Source: CAD feature listing. Evaluate the final solid. Frame: model axes, mm. Coordinates: 2 decimals unless noted, no trailing zeros. Write each loop counter-clockwise with the first axis right and the second up, starting at its lowest first coordinate (ties: lowest second). Pieces come first, ordered by that corner, then holes. Notation, with made-up numbers: (-21, 41.5) -> (36, 41.5) arc R12 cw to (36, 51.5) -> close; hole circle Ø3 at (49.5, 80.5). An arc over 180 degrees is marked (long way). One line per item, written item: value. Start each with the question number.
1. Line query: line 1 (X direction, y = 1014, z = 7.25); line 2 (Y direction, x = -143.5, z = 4.75); line 3 (Y direction, x = -800, z = 6). Output: solid intervals per line, ascending.
2. Section query C-C, the plane x = -800. Output: boundary loops of the cut face in (y, z).
3. Section query D-D, the plane x = -462. Output: boundary loops of the cut face in (y, z), and give its area (3 significant figures).
4. Section query A-A, the plane y = 80. Output: boundary loops of the cut face in (x, z).
5. Section query B-B, the plane z = 1.5. State how many separate pieces and enclosed holes the cut face has, and give its area (3 significant figures).
Autodesk Inventor part; units mm, degrees
ref_plane "YZ Plane" through (0, 0, 0) normal (1, 0, 0) x (0, 1, 0)
ref_plane "XZ Plane" through (0, 0, 0) normal (0, 1, 0) x (-1, 0, 0)
ref_plane "XY Plane" through (0, 0, 0) normal (0, 0, 1) x (1, 0, 0)
sketch "Sketch1" plane through (0, 0, 0) normal (0, 0, 1) x (1, 0, 0)
  line L0 (0, 0) -> (0, 1910) construction
  line L1 (424.5155, 1910) -> (-415.4845, 1910)
  line L2 (-415.4845, 1910) -> (-1180, 1150)
  line L3 (-1180, 0) -> (-1180, 1150)
  line L4 (960, 0) -> (960, 1342.8524)
  line L5 (424.5155, 1910) -> (960, 1342.8524)
  circle A0 centre (0, 950) radius 265 construction
  line L6 (960, 0) -> (-1180, 0)
  circle A1 centre (-1701.6377, -269.2167) radius 188.5 construction
  circle A2 centre (-800, 80) radius 55.5
  circle A3 centre (0, 950) radius 170
  line L7 (0, 1215) -> (0, 1120) construction
  line L8 (-721.2646, 955) -> (721.2646, 955) construction
  line L9 (-169.9265, 955) -> (-174.9265, 955) construction
  line L10 (-174.9265, 960) -> (-174.9265, 950)
  line L11 (-174.9265, 960) -> (-169.7056, 960)
  line L12 (-174.9265, 950) -> (-170, 950)
  line L13 (169.9265, 955) -> (174.9265, 955) construction
  line L14 (174.9265, 960) -> (174.9265, 950)
  line L15 (169.7056, 960) -> (174.9265, 960)
  line L16 (174.9265, 950) -> (170, 950)
  line L17 (-174.9265, 970) -> (174.9265, 970)
  line L18 (174.9265, 970) -> (174.9265, 940)
  line L19 (174.9265, 940) -> (-174.9265, 940)
  line L20 (-174.9265, 940) -> (-174.9265, 970)
  arc A4 (-2.4999, 780.0184) -> (2.4999, 780.0184) centre (0, 780) ccw
  arc A5 (2.4999, 1119.9816) -> (-2.4999, 1119.9816) centre (0, 1120) ccw
  point P0 (0, 955)
  point P1 (-169.7056, 940)
  point P2 (169.7056, 940)
  point P3 (168.8194, 970)
  point P4 (-168.8194, 970)
  dimension "d52" = 530
  dimension "d72" = 340
  dimension "d1" = 840
  dimension "d3" = 1150
  dimension "d12" = 1180
  dimension "d13" = 950
  dimension "d14" = 111
  dimension "d15" = 1910
  dimension "d17" = -521.6377
  dimension "d18" = 377
  dimension "d19" = -269.2167
  dimension "d34" = 380
  dimension "d35" = 80
  dimension "d37" = 2140
  dimension "d53" = 5
  dimension "d54" = 10
  dimension "d55" = 30
  dimension "d67" = 5
  dimension "d68" = 5
  dimension "d69" = 780
  dimension "d71" = 1078
extrude "Extrusion1" add sketch "Sketch1" along normal blind 10 contours L5 L4 L6 L3 L2 L1 | A3 L19 L17 | L16 L18 L19 A3 | A3 L15 L14 L16 | A3 L17 L18 L15 | L19 L20 L12 A3 | A3 L11 L20 L17 | L12 L10 L11 A3
fillet "Fillet1" radius 10 4 edges at (-168.8194, 970, 5) (-169.7056, 940, 5) (168.8194, 970, 5) (169.7056, 940, 5)
sketch "Sketch4" plane through (0, 0, 0) normal (0, 0, 1) x (1, 0, 0)
  circle A0 centre (-51.6989, 1209.9081) radius 6.5
  arc A1 (-2.4999, 1119.9816) -> (-166.985, 981.875) centre (0, 950) ccw
  line L0 (0, 950) -> (0, 1196.7062) construction
  line L1 (-51.6989, 1209.9081) -> (0, 950) construction
  point P0 (0, 0)
  point P1 (-5, 1149.9375)
  dimension "d59" = 265
  dimension "d60" = 13
  dimension "d61" = 11.25
extrude "Extrusion4" [suppressed]
pattern_circular "Circular Pattern3" [suppressed]
properties part number "ДМФ 011 Стенка_Корма"
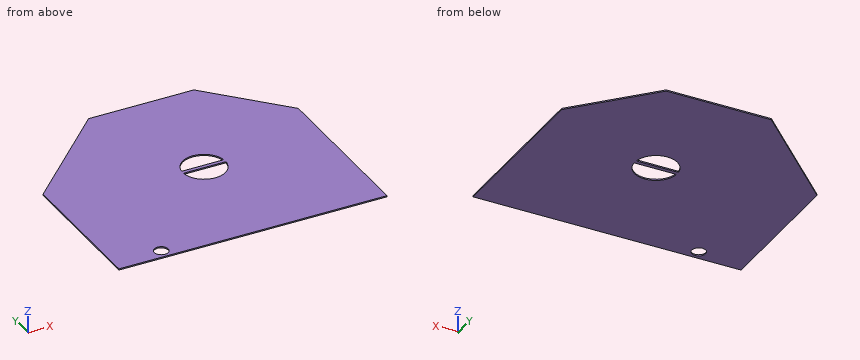
Computed values:
1. line 1: x = -1180 to -157.49, 157.49 to 960
1. line 2: y = 0 to 858.85, 940 to 970, 1041.15 to 1910
1. line 3: y = 0 to 24.5, 135.5 to 1527.76
2. outline: (0, 0) -> (24.5, 0) -> (24.5, 10) -> (0, 10) -> close; (135.5, 0) -> (1527.76, 0) -> (1527.76, 10) -> (135.5, 10) -> close
3. outline: (0, 0) -> (1863.76, 0) -> (1863.76, 10) -> (0, 10) -> close
3. area: 18,600 mm²
4. outline: (-1180, 0) -> (-855.5, 0) -> (-855.5, 10) -> (-1180, 10) -> close; (-744.5, 0) -> (960, 0) -> (960, 10) -> (-744.5, 10) -> close
5. separate pieces: 1
5. enclosed holes: 3
5. area: 3,550,000 mm²
